from build123d import *

# Parameters (mm, degrees)
F0_W     = 117.475
F0_H     = 88.9
F1_DEPTH = 15.875
F2_T     = -2.54
F3_W     = 60.325
F3_H     = 0.635
F4_DEPTH = 13.335


with BuildPart() as f1:
    # F0 (on Front) → F1 (new body)
    with BuildSketch(Plane.XZ):
        with Locations((-58.7375, -44.45)):
            Rectangle(F0_W, F0_H)
    extrude(amount=F1_DEPTH)

    # F2
    f2_openings = [f1.faces().sort_by_distance(p)[0] for p in [
        (-58.7375, 0, -44.45),
        (-58.7375, -7.9375, 0),
    ]]
    offset(amount=F2_T, openings=f2_openings)

    # F3 (on Front) → F4 (join, through all)
    with BuildSketch(Plane.XZ):
        with Locations((-84.7725, -0.3175)):
            Rectangle(F3_W, F3_H)
    extrude(amount=F4_DEPTH)


solid = f1.part
Could you check a few things on this model? Use its own coordinates, in mm. A direction names the side the tool comes from. Give positions to 0.01 mm unless a question says otherwise; leave off trailing zeros. Order: outer loops, then holes, each group sorted by start corner. A loop starts at its lowest first (then second) coordinate and runs counter-clockwise, first axis right, second up. Notation, with made-up numbers: (38.25, -4) -> (91.25, -4) arc R19 ccw to (91.25, 33) -> close; hole circle Ø1 at (-31, 11.25). An arc over 180 degrees is marked (long way). Answer in a Markdown table with one row per item. Add a question column.
Item 1: Imagine slicing it at A-A (x = -58). List the corners of the cut face in (y, z) for me (3 decimals).
Item 2: Please list where these lines run through material, in increasing order: probe 1 along Z at (x, y) = (-77, -8) (3 decimals); probe 2 along X at (y, z) = (-11.5, -77) (3 decimals); probe 3 along Y at (x, z) = (-21.5, -74.5) (3 decimals).
Item 3: Imagine slicing it at C-C (y = -2). List the corners of the cut face in (x, z) for me (3 decimals).
Item 4: Imagine slicing it at B-B (z = -16.5). List the corners of the cut face in (x, y) for me (3 decimals).
Item 5: For faces 1 (the flat face through (-114.935, -7, -44)), 2 (the flat face through (-117.475, -8, -45)), 3 (the flat face through (-2.54, -7, -44)), which set-ups out of +Z, -Z, +X, -X, +Y, -Y let a thin tool reach every point of the face, with its end or its side?
Item 6: We'd pull the mould along Z, two halves only. Please class faces 4 (the flat face through (-60, -13.335, -43)), 5 (the flat face through (-60, -8, -88.9)), 6 (the flat face through (-60, -15.875, -44)): pulls with the +Z half, pulls with the -Z half, needs draft (parallel to the pull), parting line crosses it, or undercut.
Item 7: I'm going to push flat-ended pins straight in: P1, Ø4, axis at x = -28.5, y = -2.5, coming from the +Z side; P2, Ø10, axis at x = -95, z = -19, coming from the +Y side (3 decimals); P3, Ø2, axis at x = -68, y = -6.5, coming from the +Z side. Where does each tip first touch, or does it pass through?
Item 8: Imagine slicing it at D-D (x = -10.5). List the corners of the cut face in (y, z) for me (3 decimals), and give its area (3 significant figures).
Result:
| question | item | result |
|---|---|---|
| 1 | outline | (-15.875, -88.9) -> (0, -88.9) -> (0, -86.36) -> (-13.335, -86.36) -> (-13.335, -0.635) -> (0, -0.635) -> (0, 0) -> (-15.875, 0) -> close |
| 2 | probe 1 | -88.9 to -86.36, -0.635 to 0 |
| 2 | probe 2 | -117.475 to -114.935, -2.54 to 0 |
| 2 | probe 3 | -15.875 to -13.335 |
| 3 | outline | (-117.475, -88.9) -> (0, -88.9) -> (0, 0) -> (-2.54, 0) -> (-2.54, -86.36) -> (-114.935, -86.36) -> (-114.935, -0.635) -> (-54.61, -0.635) -> (-54.61, 0) -> (-117.475, 0) -> close |
| 4 | outline | (-117.475, -15.875) -> (0, -15.875) -> (0, 0) -> (-2.54, 0) -> (-2.54, -13.335) -> (-114.935, -13.335) -> (-114.935, 0) -> (-117.475, 0) -> close |
| 5 | face 1 | +Y |
| 5 | face 2 | +Z, -Z, -X, +Y, -Y |
| 5 | face 3 | +Z, +Y |
| 6 | face 4 | undercut |
| 6 | face 5 | pulls with the -Z half |
| 6 | face 6 | needs draft |
| 7 | P1 | z = -86.36 |
| 7 | P2 | y = -13.335 |
| 7 | P3 | z = 0 |
| 8 | outline | (-15.875, -88.9) -> (0, -88.9) -> (0, -86.36) -> (-13.335, -86.36) -> (-13.335, 0) -> (-15.875, 0) -> close |
| 8 | area | 260 mm2 |
